Here's how the part is built. I have some questions about the finished solid (model axes, mm). A direction names the side the tool comes from. Coordinates: 2 decimals unless noted, no trailing zeros. Loops run counter-clockwise (first coordinate to the right, second up) from the corner with the lowest first, then second, coordinate; pieces in that order, holes last.
from build123d import *

# Parameters (mm, degrees)
SKETCH1_R           = 22.5
SKETCH1_R_2         = 6
BOSS_EXTRUDE1_DEPTH = 7
SKETCH2_R           = 8
CUT_EXTRUDE1_DEPTH  = 5
SKETCH3_R           = 1.75
CUT_EXTRUDE2_DEPTH  = 33.580669115


with BuildPart() as part:
    # Sketch1 → Boss-Extrude1 (new body)
    with BuildSketch(Plane.XY):
        Circle(SKETCH1_R)
        Circle(SKETCH1_R_2, mode=Mode.SUBTRACT)
    extrude(amount=BOSS_EXTRUDE1_DEPTH)

    # Sketch2 → Cut-Extrude1 (cut)
    with BuildSketch(Plane.XY.offset(7)):
        Circle(SKETCH2_R)
    extrude(amount=-CUT_EXTRUDE1_DEPTH, mode=Mode.SUBTRACT)

    # Sketch3 → Cut-Extrude2 (cut, through all)
    with BuildSketch(Plane.XY.offset(7)):
        with Locations((-12, 12)):
            Circle(SKETCH3_R)
        with Locations(Location((12, 12, 0), (0, 0, 180))):
            Circle(SKETCH3_R)
        with Locations((12, -12)):
            Circle(SKETCH3_R)
        with Locations(Location((-12, -12, 0), (0, 0, 180))):
            Circle(SKETCH3_R)
    extrude(amount=-CUT_EXTRUDE2_DEPTH, mode=Mode.SUBTRACT)


solid = part.part
Q1. Suppose I cut it at C-C on z = 3. Write out the boundary of the cut face in (x, y).
Q2. Please list where these lines run through material, in increasing order: probe 1 along X at (y, z) = (13, 6.25); probe 2 along Y at (x, z) = (12, 2.75).
Q3. We'd pull the mould along X, two halves only. Please class faces 1 (the cylindrical face through (12.9, -10.5, 3.5)), 2 (the cylindrical face through (-6, 0, 1)), 3 (the flat face through (5, -5, 0)), 4 (the cylindrical face through (10.382, -19.961, 3.451)): pulls with the +X half, pulls with the -X half, needs draft (parallel to the pull), parting line crosses it, or undercut.
Q4. Will these pins go through, and if not, where does the flat tip stop? P1, Ø3, axis at y = -3.5, z = 5.5, coming from the +X side; P2, Ø2, axis at y = -14, z = 4, coming from the +X side.
Q5. Suppose I cut it at D-D on y = 12. Write out the boundary of the cut face in (x, z).
Q6. Suppose I cut it at A-A on y = 0. Write out the boundary of the cut face in (x, z).
Q7. For faces 5 (the cylindrical face through (11.1, 10.5, 3.5)), 6 (the cylindrical face through (-1.73, -7.81, 4.54)), which set-ups out of +Z, -Z, +X, -X, +Y, -Y let a thin tool reach every point of the face, with its end or its side?
Check values:
1. outline: circle Ø45 at (0, 0); hole circle Ø3.5 at (-12, -12); hole circle Ø3.5 at (-12, 12); hole circle Ø16 at (0, 0); hole circle Ø3.5 at (12, -12); hole circle Ø3.5 at (12, 12)
2. probe 1: x = -18.36 to -13.44, -10.56 to 10.56, 13.44 to 18.36
2. probe 2: y = -19.03 to -13.75, -10.25 to 10.25, 13.75 to 19.03
3. face 1: undercut
3. face 2: undercut
3. face 3: needs draft
3. face 4: parting line crosses it
4. P1: stops at x = 22.41
4. P2: stops at x = 18.36
5. outline: (-19.03, 0) - (-13.75, 0) - (-13.75, 7) - (-19.03, 7) - close; (-10.25, 0) - (10.25, 0) - (10.25, 7) - (-10.25, 7) - close; (13.75, 0) - (19.03, 0) - (19.03, 7) - (13.75, 7) - close
6. outline: (-22.5, 0) - (-6, 0) - (-6, 2) - (-8, 2) - (-8, 7) - (-22.5, 7) - close; (6, 0) - (22.5, 0) - (22.5, 7) - (8, 7) - (8, 2) - (6, 2) - close
7. face 5: +Z, -Z
7. face 6: +Z
